```python
from build123d import *

# Parameters (mm, degrees)
PAD005_DEPTH    = 0.75
SKETCH003_W     = 70
SKETCH003_H     = 80
PAD003_DEPTH    = 27
THICKNESS_T     = 2
SKETCH005_W     = 35
SKETCH005_H     = 12.5
SKETCH005_W_2   = 17
SKETCH005_H_2   = 23
POCKET_DEPTH    = 5
CHAMFER_SIZE    = 2
SKETCH010_R     = 1.5
POCKET002_DEPTH = 5
SKETCH011_R     = 4.3
SKETCH011_R_2   = 1.45
PAD009_DEPTH    = 4.5
SKETCH012_W     = 3
SKETCH012_H     = 11
PAD010_DEPTH    = 7
SKETCH013_R     = 1.45
POCKET003_DEPTH = 5


with BuildPart() as pad005:
    # Sketch007 → Pad005 (new body, symmetric)
    with BuildSketch(Plane.XY.offset(19)):
        Polygon((-35.737, 39.45567), (-25.77877, 39.45567), (-25.77877, 49.4139), (25.77877, 49.4139), (25.77877, 39.45567), (35.737, 39.45567), (35.737, -22.04177), (25.77877, -22.04177), (25.77877, -32), (-25.77877, -32), (-25.77877, -22.04177), (-35.737, -22.04177), align=None)
    extrude(amount=PAD005_DEPTH, both=True)


with BuildPart() as chillermodule_case:
    # Sketch003 → Pad003 (new body)
    with BuildSketch(Plane.XY.offset(-6)):
        with Locations((0, 8.709674)):
            Rectangle(SKETCH003_W, SKETCH003_H)
    extrude(amount=PAD003_DEPTH)

    # Thickness
    thickness_openings = [chillermodule_case.faces().sort_by_distance(p)[0] for p in [
        (0, 8.709674, 21),
    ]]
    offset(amount=THICKNESS_T, openings=thickness_openings, kind=Kind.INTERSECTION)

    # Sketch005 → Pocket (cut)
    with BuildSketch(Plane.YZ.offset(37)):
        with Locations((-1.101604, 4.909958)):
            Rectangle(SKETCH005_W, SKETCH005_H)
        with Locations((33.258465, 8.215456)):
            Rectangle(SKETCH005_W_2, SKETCH005_H_2)
    extrude(amount=-POCKET_DEPTH, mode=Mode.SUBTRACT)

    # Chamfer
    chamfer_edges = [chillermodule_case.edges().sort_by_distance(p)[0] for p in [
        (0, -33.290326, -8),
        (37, 8.709674, -8),
        (37, -33.290326, 6.5),
        (-37, -33.290326, 6.5),
        (37, 50.709674, 6.5),
        (-37, 8.709674, -8),
        (-37, 50.709674, 6.5),
        (0, 50.709674, -8),
    ]]
    chamfer(chamfer_edges, length=CHAMFER_SIZE)

    # Cut: cut Pad005
    add(pad005.part, mode=Mode.SUBTRACT)

    # Sketch010 → Pocket002 (cut)
    with BuildSketch(Plane.XY.offset(-6)):
        with Locations((-32.1, 46.207886)):
            Circle(SKETCH010_R)
        with Locations((32.1, 46.207886)):
            Circle(SKETCH010_R)
        with Locations((32.1, -28.698038)):
            Circle(SKETCH010_R)
        with Locations((-32.1, -28.698038)):
            Circle(SKETCH010_R)
    extrude(amount=-POCKET002_DEPTH, mode=Mode.SUBTRACT)

    # Sketch011 → Pad009 (new body)
    with BuildSketch(Plane.XY.offset(-6)):
        with Locations((20.125536, -20.122694)):
            Circle(SKETCH011_R)
        with Locations((20.125536, -20.122694)):
            Circle(SKETCH011_R_2, mode=Mode.SUBTRACT)
        with Locations((-20.125536, -20.122694)):
            Circle(SKETCH011_R)
        with Locations((-20.125536, -20.122694)):
            Circle(SKETCH011_R_2, mode=Mode.SUBTRACT)
        with Locations((-20.125536, 20.122694)):
            Circle(SKETCH011_R)
        with Locations((-20.125536, 20.122694)):
            Circle(SKETCH011_R_2, mode=Mode.SUBTRACT)
        with Locations((20.125536, 20.122694)):
            Circle(SKETCH011_R)
        with Locations((20.125536, 20.122694)):
            Circle(SKETCH011_R_2, mode=Mode.SUBTRACT)
    extrude(amount=PAD009_DEPTH)

    # Sketch012 → Pad010 (new body)
    with BuildSketch(Plane.XY.offset(-6)):
        with Locations((19.14116, 33.381699)):
            Rectangle(SKETCH012_W, SKETCH012_H)
    extrude(amount=PAD010_DEPTH)

    # Sketch013 → Pocket003 (cut)
    with BuildSketch(Plane.XY.offset(-6)):
        with Locations((20.125536, 20.122694)):
            Circle(SKETCH013_R)
        with Locations((-20.125536, 20.122694)):
            Circle(SKETCH013_R)
        with Locations((-20.125536, -20.122694)):
            Circle(SKETCH013_R)
        with Locations((20.125536, -20.122694)):
            Circle(SKETCH013_R)
    extrude(amount=-POCKET003_DEPTH, mode=Mode.SUBTRACT)


solid = chillermodule_case.part
```
For this review, take the finished solid that the model builds, in its own axes (mm). A direction names the side the tool comes from. Give positions to 0.01 mm unless a question says otherwise; leave off trailing zeros. Write each loop counter-clockwise with the first axis right and the second up, starting at its lowest first coordinate (ties: lowest second). Pieces come first, ordered by that corner, then holes. Notation, with made-up numbers: M -6,51 L 53,51 A18 ccw 53,62 Z; hole C -19.75,-21 d10. An arc over 180 degrees is marked long. Answer as a JSON object with one key per item and string values. Group by question number.
Item 1: Tool access review of faces 1 (the flat face through (0, 48.71, 7)), 2 (the flat face through (36.01, -32.28, 7.31)), 3 (the flat face through (36, 33, -3.285)): name each direction out of +Z, -Z, +X, -X, +Y, -Y from which nothing blocks a thin tool from reaching the whole face with its end or side.
Item 2: Draft analysis for pull direction Y (two halves, no side actions). For faces 4 (the flat face through (0, 9, -6)), 5 (the flat face through (-36, 8, -7)), 6 (the flat face through (-35.764, -31.922, -6.604)), 7 (the cylindrical face through (15.83, -19.93, -3.78)), state which applies: +Y half, -Y half, draft (parallel to the pull), parting line (faces both ways), or undercut.
Item 3: For pin 1 Ø4 at (x, y) = (-20.13, -20.12) entering from +Z; pin 2 Ø2 at (x, y) = (23.5, 7) entering from +Z; pin 3 Ø0.6 at (x, z) = (36, 3) entering from -Y, all flat-tipped, find the tip position at first contact; note any pin that passes through.
Item 4: Consider section C-C on z = 0. Write out the cut boundary in (x, y).
Item 5: Consider section D-D on x = -4. Write out the cut boundary in (y, z), plus the area to 3 significant figures.
Item 6: Consider section A-A on x = 32.1. Write out the cut boundary in (y, z), plus the area to 3 significant figures.
Item 7: For probe 1 along Y at (x, z) = (-12, 19.25); probe 2 along X at (y, z) = (8, -4.75); probe 3 along X at (y, z) = (0.5, 19), list the stretches that pass through material, from the lowest coordinate up. Write a range as [from, to].
Item 8: Consider section B-B on y = 9.5. Write out the cut boundary in (x, z), plus the area to 3 significant figures.
Check result:
{
 "1": {"face 1": "+Z", "face 2": "+Z, -Z, +X, -Y", "face 3": "+X"},
 "2": {"face 4": "undercut", "face 5": "draft", "face 6": "-Y half", "face 7": "undercut"},
 "3": {"pin 1": "stops at z = -1.5", "pin 2": "stops at z = -6", "pin 3": "stops at y = -32.59"},
 "4": {"outline": "M -37,-31.29 L -35,-33.29 L 35,-33.29 L 37,-31.29 L 37,-18.6 L 35,-18.6 L 35,-31.29 L -35,-31.29 L -35,48.71 L 35,48.71 L 35,41.76 L 37,41.76 L 37,48.71 L 35,50.71 L -35,50.71 L -37,48.71 Z; M 17.64,27.88 L 20.64,27.88 L 20.64,38.88 L 17.64,38.88 Z; M 35,16.4 L 37,16.4 L 37,24.76 L 35,24.76 Z"},
 "5": {"outline": "M -33.29,-6 L -31.29,-8 L 48.71,-8 L 50.71,-6 L 50.71,21 L 48.71,21 L 48.71,19.75 L 49.41,19.75 L 49.41,18.25 L 48.71,18.25 L 48.71,-6 L -31.29,-6 L -31.29,18.25 L -32,18.25 L -32,19.75 L -31.29,19.75 L -31.29,21 L -33.29,21 Z", "area": "270 mm^2"},
 "6": {"outline": "M -33.29,-6 L -31.29,-8 L -30.2,-8 L -30.2,-6 L -31.29,-6 L -31.29,21 L -33.29,21 Z; M -27.2,-8 L 44.71,-8 L 44.71,-6 L -27.2,-6 Z; M 47.71,-8 L 48.71,-8 L 50.71,-6 L 50.71,21 L 48.71,21 L 48.71,-6 L 47.71,-6 Z", "area": "260 mm^2"},
 "7": {"probe 1": "y = [-33.29, -32], [49.41, 50.71]", "probe 2": "x = [-37, -35], [35, 37]", "probe 3": "x = [-37, -35.74], [35.74, 37]"},
 "8": {"outline": "M -37,-6 L -35,-8 L 35,-8 L 37,-6 L 37,-1.34 L 35,-1.34 L 35,-6 L -35,-6 L -35,18.25 L -35.74,18.25 L -35.74,19.75 L -35,19.75 L -35,21 L -37,21 Z; M 35,11.16 L 37,11.16 L 37,21 L 35,21 L 35,19.75 L 35.74,19.75 L 35.74,18.25 L 35,18.25 Z", "area": "225 mm^2"}
}
